from build123d import *

# Parameters (mm, degrees)
SKETCH1_W           = 88.9
SKETCH1_H           = 88.9
BOSS_EXTRUDE1_DEPTH = 12.7
SKETCH2_OUTSIDE_W   = 116.172
SKETCH2_OUTSIDE_H   = 116.172
SKETCH2_OUTSIDE_W_2 = 76.2
SKETCH2_OUTSIDE_H_2 = 76.2
CUT_EXTRUDE3_DEPTH  = 6.35
SKETCH3_R           = 2.3876
CUT_EXTRUDE4_DEPTH  = 65.131856359
CHAMFER1_SIZE       = 0.635
SKETCH4_R           = 3.175
CUT_EXTRUDE5_DEPTH  = 7.62


with BuildPart() as part:
    # Sketch1 → Boss-Extrude1 (new body)
    with BuildSketch(Plane(origin=(0, 0, 0), x_dir=(1, 0, 0), z_dir=(0, 1, 0))):
        Rectangle(SKETCH1_W, SKETCH1_H)
    extrude(amount=BOSS_EXTRUDE1_DEPTH)

    # Sketch2 outside → Cut-Extrude3 (cut)
    with BuildSketch(Plane(origin=(0, 0, 0), x_dir=(1, 0, 0), z_dir=(0, 1, 0))):
        Rectangle(SKETCH2_OUTSIDE_W, SKETCH2_OUTSIDE_H)
        Rectangle(SKETCH2_OUTSIDE_W_2, SKETCH2_OUTSIDE_H_2, mode=Mode.SUBTRACT)
    extrude(amount=CUT_EXTRUDE3_DEPTH, mode=Mode.SUBTRACT)

    # Sketch3 → Cut-Extrude4 (cut, through all)
    with BuildSketch(Plane(origin=(0, 12.7, 0), x_dir=(1, 0, 0), z_dir=(0, 1, 0))):
        with Locations(Location((-31.75, 0, 0), (0, 0, 270))):
            Circle(SKETCH3_R)
    extrude(amount=-CUT_EXTRUDE4_DEPTH, mode=Mode.SUBTRACT)

    # Chamfer1
    chamfer1_edges = [part.edges().sort_by_distance(p)[0] for p in [
        (-44.45, 12.7, 0),
        (0, 12.7, 44.45),
        (44.45, 12.7, 0),
        (0, 12.7, -44.45),
    ]]
    chamfer(chamfer1_edges, length=CHAMFER1_SIZE)

    # Sketch4 → Cut-Extrude5 (cut)
    with BuildSketch(Plane.XZ):
        with Locations(Location((-31.75, 15.875, 0), (0, 0, 270))):
            Circle(SKETCH4_R)
        with Locations(Location((-31.75, -15.875, 0), (0, 0, 270))):
            Circle(SKETCH4_R)
    extrude(amount=-CUT_EXTRUDE5_DEPTH, mode=Mode.SUBTRACT)


solid = part.part
Here's how the part is built. I have some questions about the finished solid (model axes, mm). A direction names the side the tool comes from. Coordinates: 2 decimals unless noted, no trailing zeros. Loops run counter-clockwise (first coordinate to the right, second up) from the corner with the lowest first, then second, coordinate; pieces in that order, holes last.
1. I need wall thicknesses on L1, parallel to Z at x = -34.5, y = 2.25; L2, parallel to X at y = 3, z = -32.5. Which ranges of each line are inside material? Lowest first, please.
2. Imagine slicing it at D-D, the plane x = 33. Please give me the cut outline in (y, z) (3 decimals), and give its area (3 significant figures).
3. If we mould it in two halves opening along Z, with no side actions, what happens to faces 6 (the flat face through (-1, 9, 44.45)), 7 (the flat face through (-32, 7.62, 16)), 8 (the flat face through (38.1, 3, 1))? For each: pulls with the +Z half, pulls with the -Z half, needs draft (parallel to the pull), parting line crosses it, or undercut.
4. Imagine slicing it at A-A, the plane z = 0. Please give me the cut outline in (x, y) (3 decimals), and give its area (3 significant figures).
5. Imagine slicing it at B-B, the plane x = -31.75. Please give me the cut outline in (y, z) (3 decimals).
6. For faces 1 (the cylindrical face through (-29.383, 6.439, -0.311)), 2 (the flat face through (-38.1, 3, 1)), 3 (the flat face through (-32, 7.62, -16)), 4 (the flat face through (-1, 3, -38.1)), 5 (the flat face through (-1, 3, 38.1)), which set-ups out of +Z, -Z, +X, -X, +Y, -Y let a thin tool reach every point of the face, with its end or its side?
7. For P1, Ø7, axis at y = 4.5, z = -15.5, coming from the -X side; P2, Ø1.5, axis at y = 2, z = 10, coming from the +X side; P3, Ø3, axis at x = 0.5, y = 4.5, coming from the +Z side; P4, Ø3, axis at x = -30.5, z = 15, coming from the -Y side, each with a flat end and sliding along its axis, tell me the tip position at first contact or that it passes through.
8. Imagine slicing it at C-C, the plane y = 4.75. Please give me the cut outline in (x, z) (3 decimals).
Taken from the geometry:
1. L1: z = -38.1 to -17.46, -14.29 to 14.29, 17.46 to 38.1
1. L2: x = -38.1 to 38.1
2. outline: (0, -38.1) - (6.35, -38.1) - (6.35, -44.45) - (12.065, -44.45) - (12.7, -43.815) - (12.7, 43.815) - (12.065, 44.45) - (6.35, 44.45) - (6.35, 38.1) - (0, 38.1) - close
2. area: 1,050 mm2
3. face 6: pulls with the +Z half
3. face 7: undercut
3. face 8: needs draft
4. outline: (-44.45, 6.35) - (-38.1, 6.35) - (-38.1, 0) - (-34.138, 0) - (-34.138, 12.7) - (-43.815, 12.7) - (-44.45, 12.065) - close; (-29.362, 0) - (38.1, 0) - (38.1, 6.35) - (44.45, 6.35) - (44.45, 12.065) - (43.815, 12.7) - (-29.362, 12.7) - close
4. area: 987 mm2
5. outline: (0, -38.1) - (6.35, -38.1) - (6.35, -44.45) - (12.065, -44.45) - (12.7, -43.815) - (12.7, -2.388) - (0, -2.388) - (0, -12.7) - (7.62, -12.7) - (7.62, -19.05) - (0, -19.05) - close; (0, 2.388) - (12.7, 2.388) - (12.7, 43.815) - (12.065, 44.45) - (6.35, 44.45) - (6.35, 38.1) - (0, 38.1) - (0, 19.05) - (7.62, 19.05) - (7.62, 12.7) - (0, 12.7) - close
6. face 1: +Y, -Y
6. face 2: +Z, -Z, -X, -Y
6. face 3: -Y
6. face 4: -Z, +X, -X, -Y
6. face 5: +Z, +X, -X, -Y
7. P1: stops at x = -44.45
7. P2: stops at x = 38.1
7. P3: stops at z = 38.1
7. P4: stops at y = 7.62
8. outline: (-38.1, -38.1) - (38.1, -38.1) - (38.1, 38.1) - (-38.1, 38.1) - close; hole circle Ø6.35 at (-31.75, -15.875); hole circle Ø6.35 at (-31.75, 15.875); hole circle Ø4.775 at (-31.75, 0)
